The model under review builds one solid part; all positions refer to its coordinate system, in mm. A direction names the side the tool comes from. Give positions to 0.01 mm unless a question says otherwise; leave off trailing zeros. Order: outer loops, then holes, each group sorted by start corner. A loop starts at its lowest first (then second) coordinate and runs counter-clockwise, first axis right, second up. Notation, with made-up numbers: (39, 68) -> (93, 68) arc R28 ccw to (93, 95) -> close; hole circle Ø4 at (28, 58.5). An arc over 180 degrees is marked (long way). Use one line per item in the form item = value.
```python
from build123d import *

# Parameters (mm, degrees)
F1_DEPTH = 3.175
F2_R     = 3.175
F3_DEPTH = 25.4
F5_DEPTH = 1.5
F6_R     = 6
F7_DEPTH = 0.1
F8_R     = 25.33
F8_R_2   = 26.99
F9_DEPTH = 3.176


with BuildPart() as f1:
    # F0 (on Front) → F1 (new body)
    with BuildSketch(Plane.XZ):
        with BuildLine():
            Line((98.425, 98.425), (-98.425, 98.425))
            ThreePointArc((-98.425, 98.425), (-102.915128, 96.565128), (-104.775, 92.075))
            Line((-104.775, 92.075), (-104.775, -92.075))
            ThreePointArc((-104.775, -92.075), (-102.915128, -96.565128), (-98.425, -98.425))
            Line((-98.425, -98.425), (98.425, -98.425))
            ThreePointArc((98.425, -98.425), (102.915128, -96.565128), (104.775, -92.075))
            Line((104.775, -92.075), (104.775, 92.075))
            ThreePointArc((104.775, 92.075), (102.915128, 96.565128), (98.425, 98.425))
        make_face()
    extrude(amount=F1_DEPTH)

    # F2 (on face) → F3 (cut)
    with BuildSketch(Plane.XZ.offset(3.175)):
        with Locations((-98.425, 92.075)):
            Circle(F2_R)
        with Locations((98.425, 92.075)):
            Circle(F2_R)
        with Locations((98.425, -92.075)):
            Circle(F2_R)
        with Locations((-98.425, -92.075)):
            Circle(F2_R)
    extrude(amount=-F3_DEPTH, mode=Mode.SUBTRACT)

    # F4 (on face) → F5 (cut)
    with BuildSketch(Plane.XZ.offset(3.175)):
        with BuildLine():
            Line((54.84, -26.5), (-54.84, -26.5))
            ThreePointArc((-54.84, -26.5), (-63.820256, -30.219744), (-67.54, -39.2))
            ThreePointArc((-67.54, -39.2), (-63.820256, -48.180256), (-54.84, -51.9))
            Line((-54.84, -51.9), (54.84, -51.9))
            ThreePointArc((54.84, -51.9), (63.820256, -48.180256), (67.54, -39.2))
            ThreePointArc((67.54, -39.2), (63.820256, -30.219744), (54.84, -26.5))
        make_face()
    extrude(amount=-F5_DEPTH, mode=Mode.SUBTRACT)

    # F6 (on face) → F7 (cut)
    with BuildSketch(Plane.XZ.offset(3.175)):
        with Locations((-81.8, -39.2)):
            Circle(F6_R)
        with Locations((0, -77.7)):
            Circle(F6_R)
        with Locations((81.8, -39.2)):
            Circle(F6_R)
    extrude(amount=-F7_DEPTH, mode=Mode.SUBTRACT)

    # F8 (on face) → F9 (cut, through all)
    with BuildSketch(Plane.XZ.offset(3.175)):
        with Locations((-65, 43.9)):
            Circle(F8_R)
        with Locations((65, 43.9)):
            Circle(F8_R)
        with Locations((0, 43.9)):
            Circle(F8_R_2)
    extrude(amount=-F9_DEPTH, mode=Mode.SUBTRACT)


solid = f1.part
```
1. Add section B-B on y = -2.5. Count the separate pieces of the cut face and the enclosed holes in it, then the cut area to 3 significant figures.
Values:
separate_pieces = 1
enclosed_holes = 8
area = 31,500 mm^2
2. Add section C-C on z = 28. Give the boundary of the cut face in (x, y) (3 decimals).
Values:
outline = (-104.775, -3.175) -> (-84.718, -3.175) -> (-84.718, 0) -> (-104.775, 0) -> close; (-45.282, -3.175) -> (-21.809, -3.175) -> (-21.809, 0) -> (-45.282, 0) -> close; (21.809, -3.175) -> (45.282, -3.175) -> (45.282, 0) -> (21.809, 0) -> close; (84.718, -3.175) -> (104.775, -3.175) -> (104.775, 0) -> (84.718, 0) -> close
3. Add section D-D on x = 0. Give the boundary of the cut face in (y, z) (3 decimals).
Values:
outline = (-3.175, -98.425) -> (0, -98.425) -> (0, 16.91) -> (-3.175, 16.91) -> (-3.175, -26.5) -> (-1.675, -26.5) -> (-1.675, -51.9) -> (-3.175, -51.9) -> (-3.175, -71.7) -> (-3.075, -71.7) -> (-3.075, -83.7) -> (-3.175, -83.7) -> close; (-3.175, 70.89) -> (0, 70.89) -> (0, 98.425) -> (-3.175, 98.425) -> close
4. Tool access review of faces 3 (the face through (-41, -2, 52)), 4 (the face through (-1, -1.675, -39)): name each direction out of +Z, -Z, +X, -X, +Y, -Y from which nothing blocks a thin tool from reaching the whole face with its end or side.
Values:
face_3 = +Y, -Y
face_4 = -Y
5. For L1, parallel to Z at x = 0, y = -2.45 (3 decimals); L2, parallel to X at y = -1, z = 23.5 (3 decimals); L3, parallel to Z at x = 56, y = -2.55 (3 decimals), list the stretches that pass through material, from the lowest coordinate up.
Values:
L1 = -98.425 to -51.9, -26.5 to 16.91, 70.89 to 98.425
L2 = -104.775 to -80.015, -49.985 to -17.672, 17.672 to 49.985, 80.015 to 104.775
L3 = -98.425 to -51.847, -26.553 to 20.223, 67.577 to 98.425
6. The part is to be moulded in two halves that separate along Z. For faces 1 (the face through (-102.87, -1.57, 96.61)), 2 (the face through (-99.113, -1.61, -95.174)), say which applies: +Z half, -Z half, draft (parallel to the pull), parting line (faces both ways), or undercut.
Values:
face_1 = +Z half
face_2 = undercut
7. For pin 1 Ø3.5 at (x, z) = (83, -37.5) entering from -Y (3 decimals); pin 2 Ø20.5 at (x, z) = (-24.5, -39.5) entering from -Y (3 decimals), all flat-tipped, find the tip position at first contact; note any pin that passes through.
Values:
pin_1 = -3.075
pin_2 = -1.675
8. Add section A-A on x = 65. Give the boundary of the cut face in (y, z) (3 decimals), then the cut area to 3 significant figures.
Values:
outline = (-3.175, -98.425) -> (0, -98.425) -> (0, 18.57) -> (-3.175, 18.57) -> (-3.175, -31.58) -> (-1.675, -31.58) -> (-1.675, -46.82) -> (-3.175, -46.82) -> close; (-3.175, 69.23) -> (0, 69.23) -> (0, 98.425) -> (-3.175, 98.425) -> close
area = 441 mm^2
